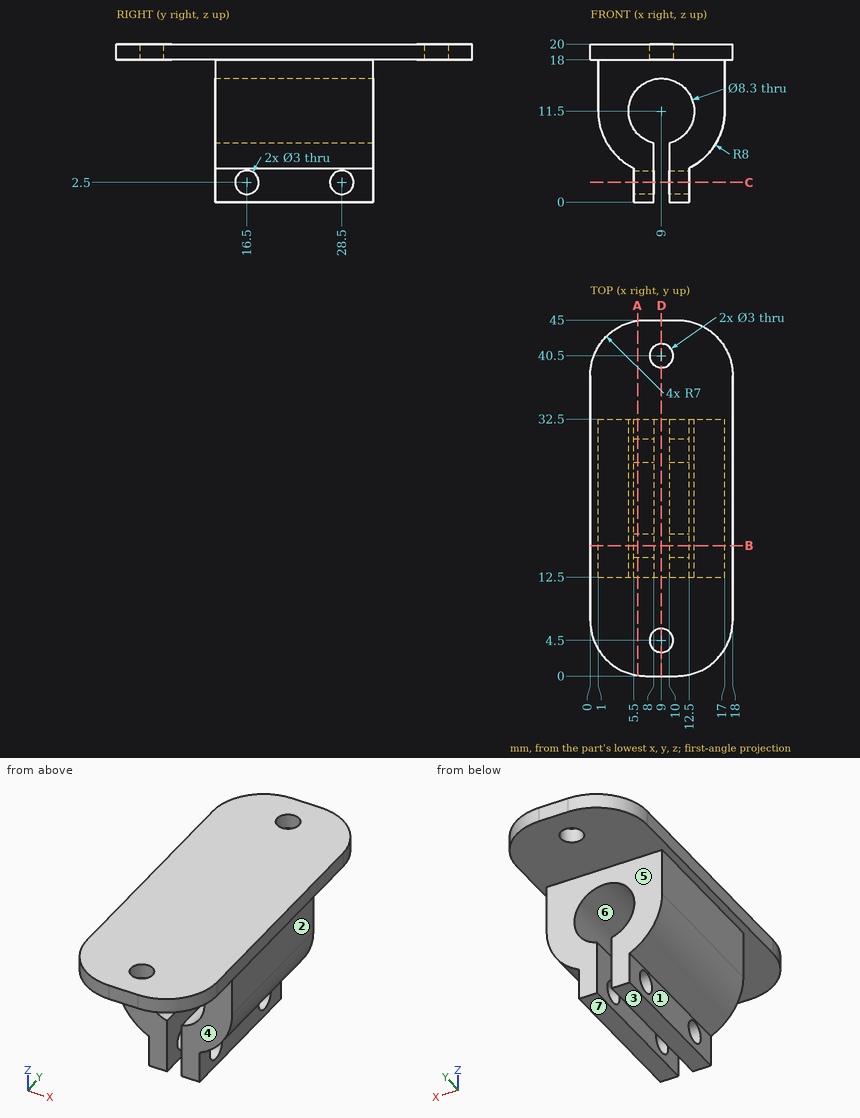
Check sheet for the drawn part. Datum: minimum x, y, z corner. Units: mm. A direction names the side the tool comes from. Round coordinates to 2 decimals unless told otherwise and drop trailing zeros. Order: outer loops, then holes, each group sorted by start corner. A loop starts at its lowest first (then second) coordinate and runs counter-clockwise, first axis right, second up.
(1) Cross-section at C-C, the plane z = 2.5. Enter the section's corners in (x, y), and give its area (3 significant figures).
(2) Cross-section at B-B, the plane y = 16.5. Enter the section's corners in (x, z), and give its area (3 significant figures).
(3) Cross-section at D-D, the plane x = 9. Enter the section's corners in (y, z), and give its area (3 significant figures).
(4) Access from +Z, -Z, +X, -X, +Y, -Y to the whole of each face (thin tool, end or side, straight path). Record for the marked faces 1, 2, 3 and 4.
(5) Draft check along Z on the marked faces 5, 6 and 7. Enter one of: pulls with the +Z half, pulls with the -Z half, needs draft (parallel to the pull), parting line crosses it, or undercut.
(6) Go/stop test with flat-tipped pins: P1, Ø5, axis at x = 7.5, z = 13.5, coming from the -Y side; P2, Ø5, axis at y = 16.5, z = 2.5, coming from the +X side; P3, Ø2, axis at y = 25.5, z = 2, coming from the +X side; P4, Ø2.5, axis at y = 28.5, z = 2.5, coming from the -X side. Record where each tip stops, or that it passes through.
(7) Scan lines: probe 1 along Y at (x, z) = (9, 19.4); probe 2 along Z at (x, y) = (17.25, 16); probe 3 along Y at (x, z) = (2.25, 17). Record each from-to range of solid material in increasing order.
(8) Cross-section at A-A, the plane x = 6. Enter the section's corners in (y, z).
Check sheet entries:
1. outline: (5.5, 12.5) - (8, 12.5) - (8, 15) - (5.5, 15) - close; (5.5, 18) - (8, 18) - (8, 27) - (5.5, 27) - close; (5.5, 30) - (8, 30) - (8, 32.5) - (5.5, 32.5) - close; (10, 12.5) - (12.5, 12.5) - (12.5, 15) - (10, 15) - close; (10, 18) - (12.5, 18) - (12.5, 27) - (10, 27) - close; (10, 30) - (12.5, 30) - (12.5, 32.5) - (10, 32.5) - close
1. area: 70.0 mm2
2. outline: (0, 18) - (1, 18) - (1, 11.5) arc R8 ccw to (5.5, 4.31) - (5.5, 4) - (8, 4) - (8, 7.47) arc R4.15 cw (long way) to (10, 7.47) - (10, 4) - (12.5, 4) - (12.5, 4.31) arc R8 ccw to (17, 11.5) - (17, 18) - (18, 18) - (18, 20) - (0, 20) - close; (5.5, 0) - (8, 0) - (8, 1) - (5.5, 1) - close; (10, 0) - (12.5, 0) - (12.5, 1) - (10, 1) - close
2. area: 183 mm2
3. outline: (0, 18) - (3, 18) - (3, 20) - (0, 20) - close; (6, 18) - (12.5, 18) - (12.5, 15.65) - (32.5, 15.65) - (32.5, 18) - (39, 18) - (39, 20) - (6, 20) - close; (42, 18) - (45, 18) - (45, 20) - (42, 20) - close
3. area: 125 mm2
4. face 1: -Z, -X, +Y, -Y
4. face 2: -Z, +X, +Y, -Y
4. face 3: -Z, +X, -X, +Y, -Y
4. face 4: -Z, +X, -X, -Y
5. face 5: needs draft
5. face 6: undercut
5. face 7: pulls with the -Z half
6. P1: stops at y = 12.5
6. P2: stops at x = 13.66
6. P3: stops at x = 12.5
6. P4: passes through
7. probe 1: y = 0 to 3, 6 to 39, 42 to 45
7. probe 2: z = 18 to 20
7. probe 3: y = 12.5 to 32.5
8. outline: (0.07, 18) - (12.5, 18) - (12.5, 14.37) - (32.5, 14.37) - (32.5, 18) - (44.93, 18) - (44.93, 20) - (0.07, 20) - close; (12.5, 0) - (32.5, 0) - (32.5, 8.63) - (12.5, 8.63) - close; hole circle Ø3 at (16.5, 2.5); hole circle Ø3 at (28.5, 2.5)
